from build123d import *

# Parameters (mm, degrees)
BOSS_EXTRUDE1_DEPTH = 100
CHAMFER1_SIZE       = 2


with BuildPart() as part:
    # Sketch2 → Boss-Extrude1 (new body)
    with BuildSketch(Plane.XY):
        Polygon((-50, 0), (50, 0), (50, 5.5), (27, 5.5), (27, 10), (16, 10), (16, 8), (-16, 8), (-16, 10), (-27, 10), (-27, 5.5), (-50, 5.5), align=None)
    extrude(amount=BOSS_EXTRUDE1_DEPTH)

    # Chamfer1
    chamfer1_edges = [part.edges().sort_by_distance(p)[0] for p in [
        (-50, 2.75, 0),
        (50, 2.75, 0),
        (-50, 2.75, 100),
        (50, 2.75, 100),
    ]]
    chamfer(chamfer1_edges, length=CHAMFER1_SIZE)


solid = part.part
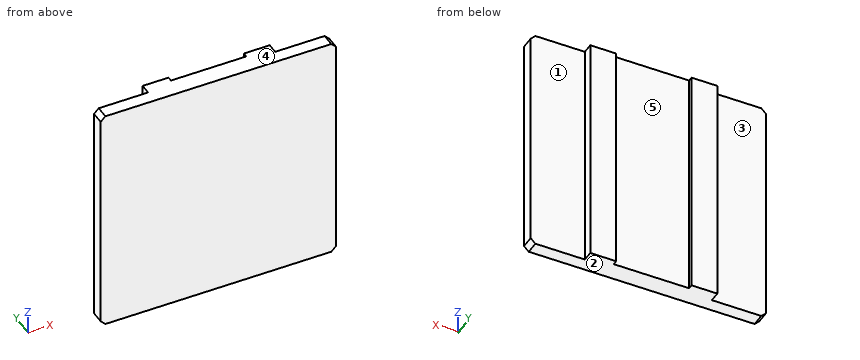
Can you work these out from the model? Positions are in its coordinate system, mm. Face numbers are marked on the shaded views. A direction names the side the tool comes from. Round coordinates to 2 decimals unless told otherwise and drop trailing zeros. Loops run counter-clockwise (first coordinate to the right, second up) from the corner with the lowest first, then second, coordinate; pieces in that order, holes last. Notation, with made-up numbers: (-7.75, -22.5) - (41.25, -22.5) arc R27 ccw to (41.25, 13.5) - close; hole circle Ø7 at (19.25, 57). An arc over 180 degrees is marked (long way). Answer in a Markdown table with one row per item. Add a question column.
Q1. For pin 1 Ø11.5 at (x, z) = (38.5, 40) entering from +Y; pin 2 Ø3.5 at (y, z) = (8.5, 26.5) entering from -X; pin 3 Ø2 at (y, z) = (8.5, 39.5) entering from +X, each with a flat end and sliding along its axis, tell me the tip position at first contact or that it passes through.
Q2. I need wall thicknesses on L1, parallel to Y at x = -28, z = 40; L2, parallel to X at y = 6, z = 43; L3, parallel to Y at x = -3, z = 65. Which ranges of each line are inside material? Lowest first, please.
Q3. I want a section at A-A on z = 50. List the corners of the cut face in (x, y) for me.
Q4. We'd pull the mould along X, two halves only. Please class the marked faces 4 and 5: pulls with the +X half, pulls with the -X half, needs draft (parallel to the pull), parting line crosses it, or undercut.
Q5. I want a section at C-C on x = -1.5. List the corners of the cut face in (y, z) for me, and give its area (3 significant figures).
Q6. Which directions (+Z, -Z, +X, -X, +Y, -Y) give clear straight access to the entire face, cutting with the end or side of a thin tool? Please do the marked faces 1, 2 and 3.
Q7. I want a section at B-B on x = 43.5. List the corners of the cut face in (y, z) for me.
A:
| question | item | result |
|---|---|---|
| 1 | pin 1 | y = 5.5 |
| 1 | pin 2 | x = -27 |
| 1 | pin 3 | x = 27 |
| 2 | L1 | 0 to 5.5 |
| 2 | L2 | -27 to 27 |
| 2 | L3 | 0 to 8 |
| 3 | outline | (-50, 0) - (50, 0) - (50, 5.5) - (27, 5.5) - (27, 10) - (16, 10) - (16, 8) - (-16, 8) - (-16, 10) - (-27, 10) - (-27, 5.5) - (-50, 5.5) - close |
| 4 | face 4 | needs draft |
| 4 | face 5 | undercut |
| 5 | outline | (0, 0) - (8, 0) - (8, 100) - (0, 100) - close |
| 5 | area | 800 mm^2 |
| 6 | face 1 | +Z, -Z, +X, +Y |
| 6 | face 2 | -Z, +X, -X, +Y, -Y |
| 6 | face 3 | +Z, -Z, -X, +Y |
| 7 | outline | (0, 0) - (5.5, 0) - (5.5, 100) - (0, 100) - close |
